from build123d import *

# Parameters (mm, degrees)
F1_DEPTH = 5
F3_D     = 5.1
F4_R     = 2.1
F5_DEPTH = 25


with BuildPart() as f1:
    # F0 (on Top) → F1 (new body)
    with BuildSketch(Plane.XY):
        Polygon((84.6812899327, 58.5268347502), (-92.3187100673, 58.5268347502), (-92.3187100673, 8.5268347502), (-44.3187100673, 8.5268347502), (36.6812899327, 8.5268347502), (84.6812899327, 8.5268347502), align=None)
    extrude(amount=F1_DEPTH)

    # F3 (through all)
    with Locations(Plane.XY.offset(5)):
        with Locations((-10.8187100673, 27.5268347502), (-3.8187100673, 48.5268347502), (3.1812899327, 27.5268347502), (-3.8187100673, 15.2268347502)):
            Hole(F3_D / 2)

    # F4 (on face) → F5 (cut)
    with BuildSketch(Plane.XY.offset(5)):
        with Locations((-63.3187100673, -6.4731652498)):
            Circle(F4_R)
        with Locations((55.6812899327, -14.4731652498)):
            Circle(F4_R)
        with Locations((-83.3187100673, -14.4731652498)):
            Circle(F4_R)
        with Locations((-73.3187100673, -43.9731652498)):
            Circle(F4_R)
        with Locations((75.6812899327, -6.4731652498)):
            Circle(F4_R)
        with Locations((65.6812899327, -43.9731652498)):
            Circle(F4_R)
    extrude(amount=-F5_DEPTH, mode=Mode.SUBTRACT)


solid = f1.part
Source: CAD feature listing. Evaluate the final solid. Frame: model axes, mm. Round coordinates to 2 decimals unless told otherwise and drop trailing zeros. Answer as CSV lines item,"result".
Q1. Contact query for a flat-ended pin moving along its axis: pin 1 (6 mm diameter, centred on x = 9.5, y = 14, fed in from -Z). Output: stop coordinate, or through.
Verdict:
pin 1,"stops at z = 0"
Q2. Pull-direction query (X, two-part tool) for faces 1 (the face through (-4.995, 12.965, 2.465)), 2 (the face through (84.681, 33, 2)), 3 (the face through (-92.319, 34, 2)), 4 (the face through (-5, 34, 5)); classes: +X half, -X half, draft (parallel to the pull), parting line (faces both ways), or undercut.
Verdict:
face 1,"undercut"
face 2,"+X half"
face 3,"-X half"
face 4,"draft"
Q3. Line query: line 1 along X through (y, z) = (28.5, 0.4); line 2 along X through (y, z) = (25.5, 0.4); line 3 along X through (y, z) = (46.5, 2.75). Output: solid intervals per line, ascending.
Verdict:
line 1,"x = -92.32 to -13.18, -8.46 to 0.82, 5.54 to 84.68"
line 2,"x = -92.32 to -12.37, -9.27 to 1.63, 4.73 to 84.68"
line 3,"x = -92.32 to -5.37, -2.27 to 84.68"
